```python
from build123d import *

# Parameters (mm, degrees)
BOSS_EXTRUDE1_DEPTH = 3.175
CUT_EXTRUDE1_REACH  = 116.795
SKETCH2_R           = 1.5875


with BuildPart() as part:
    # Sketch1 → Boss-Extrude1 (new body)
    with BuildSketch(Plane.XY):
        Polygon((0, 0), (0, 53.34), (-101.6, 53.34), (-87.988181024, -50.8), align=None)
    extrude(amount=BOSS_EXTRUDE1_DEPTH)

    # Sketch2 → Cut-Extrude1 (cut, up to next)
    with BuildSketch(Plane(origin=(0, 0, 0), x_dir=(-1, 0, 0), z_dir=(0, 0, -1)), mode=Mode.PRIVATE) as cut_extrude1_sk1:
        with Locations((12.7, 40.64)):
            Circle(SKETCH2_R)
    cut_extrude1_tool1 = extrude(cut_extrude1_sk1.sketch, amount=-CUT_EXTRUDE1_REACH, mode=Mode.PRIVATE) & part.part
    # Sketch2 → Cut-Extrude1 (cut, up to next)
    with BuildSketch(Plane(origin=(0, 0, 0), x_dir=(-1, 0, 0), z_dir=(0, 0, -1)), mode=Mode.PRIVATE) as cut_extrude1_sk2:
        with Locations((31.75, 40.64)):
            Circle(SKETCH2_R)
    cut_extrude1_tool2 = extrude(cut_extrude1_sk2.sketch, amount=-CUT_EXTRUDE1_REACH, mode=Mode.PRIVATE) & part.part
    # Sketch2 → Cut-Extrude1 (cut, up to next)
    with BuildSketch(Plane(origin=(0, 0, 0), x_dir=(-1, 0, 0), z_dir=(0, 0, -1)), mode=Mode.PRIVATE) as cut_extrude1_sk3:
        with Locations((50.8, 40.64)):
            Circle(SKETCH2_R)
    cut_extrude1_tool3 = extrude(cut_extrude1_sk3.sketch, amount=-CUT_EXTRUDE1_REACH, mode=Mode.PRIVATE) & part.part
    # Sketch2 → Cut-Extrude1 (cut, up to next)
    with BuildSketch(Plane(origin=(0, 0, 0), x_dir=(-1, 0, 0), z_dir=(0, 0, -1)), mode=Mode.PRIVATE) as cut_extrude1_sk4:
        with Locations((69.85, 40.64)):
            Circle(SKETCH2_R)
    cut_extrude1_tool4 = extrude(cut_extrude1_sk4.sketch, amount=-CUT_EXTRUDE1_REACH, mode=Mode.PRIVATE) & part.part
    # Sketch2 → Cut-Extrude1 (cut, up to next)
    with BuildSketch(Plane(origin=(0, 0, 0), x_dir=(-1, 0, 0), z_dir=(0, 0, -1)), mode=Mode.PRIVATE) as cut_extrude1_sk5:
        with Locations((88.9, 40.64)):
            Circle(SKETCH2_R)
    cut_extrude1_tool5 = extrude(cut_extrude1_sk5.sketch, amount=-CUT_EXTRUDE1_REACH, mode=Mode.PRIVATE) & part.part
    # Sketch2 → Cut-Extrude1 (cut, up to next)
    with BuildSketch(Plane(origin=(0, 0, 0), x_dir=(-1, 0, 0), z_dir=(0, 0, -1)), mode=Mode.PRIVATE) as cut_extrude1_sk6:
        with Locations((11.903880744, 8.025962948)):
            Circle(SKETCH2_R)
    cut_extrude1_tool6 = extrude(cut_extrude1_sk6.sketch, amount=-CUT_EXTRUDE1_REACH, mode=Mode.PRIVATE) & part.part
    # Sketch2 → Cut-Extrude1 (cut, up to next)
    with BuildSketch(Plane(origin=(0, 0, 0), x_dir=(-1, 0, 0), z_dir=(0, 0, -1)), mode=Mode.PRIVATE) as cut_extrude1_sk7:
        with Locations((28.401664686, -1.499037052)):
            Circle(SKETCH2_R)
    cut_extrude1_tool7 = extrude(cut_extrude1_sk7.sketch, amount=-CUT_EXTRUDE1_REACH, mode=Mode.PRIVATE) & part.part
    # Sketch2 → Cut-Extrude1 (cut, up to next)
    with BuildSketch(Plane(origin=(0, 0, 0), x_dir=(-1, 0, 0), z_dir=(0, 0, -1)), mode=Mode.PRIVATE) as cut_extrude1_sk8:
        with Locations((44.899448628, -11.024037052)):
            Circle(SKETCH2_R)
    cut_extrude1_tool8 = extrude(cut_extrude1_sk8.sketch, amount=-CUT_EXTRUDE1_REACH, mode=Mode.PRIVATE) & part.part
    # Sketch2 → Cut-Extrude1 (cut, up to next)
    with BuildSketch(Plane(origin=(0, 0, 0), x_dir=(-1, 0, 0), z_dir=(0, 0, -1)), mode=Mode.PRIVATE) as cut_extrude1_sk9:
        with Locations((61.39723257, -20.549037052)):
            Circle(SKETCH2_R)
    cut_extrude1_tool9 = extrude(cut_extrude1_sk9.sketch, amount=-CUT_EXTRUDE1_REACH, mode=Mode.PRIVATE) & part.part
    # Sketch2 → Cut-Extrude1 (cut, up to next)
    with BuildSketch(Plane(origin=(0, 0, 0), x_dir=(-1, 0, 0), z_dir=(0, 0, -1)), mode=Mode.PRIVATE) as cut_extrude1_sk10:
        with Locations((77.895016512, -30.074037052)):
            Circle(SKETCH2_R)
    cut_extrude1_tool10 = extrude(cut_extrude1_sk10.sketch, amount=-CUT_EXTRUDE1_REACH, mode=Mode.PRIVATE) & part.part
    add(cut_extrude1_tool1.solids().sort_by_distance((-12.7, 40.64, 0))[0], mode=Mode.SUBTRACT)
    add(cut_extrude1_tool2.solids().sort_by_distance((-31.75, 40.64, 0))[0], mode=Mode.SUBTRACT)
    add(cut_extrude1_tool3.solids().sort_by_distance((-50.8, 40.64, 0))[0], mode=Mode.SUBTRACT)
    add(cut_extrude1_tool4.solids().sort_by_distance((-69.85, 40.64, 0))[0], mode=Mode.SUBTRACT)
    add(cut_extrude1_tool5.solids().sort_by_distance((-88.9, 40.64, 0))[0], mode=Mode.SUBTRACT)
    add(cut_extrude1_tool6.solids().sort_by_distance((-11.903881, 8.025963, 0))[0], mode=Mode.SUBTRACT)
    add(cut_extrude1_tool7.solids().sort_by_distance((-28.401665, -1.499037, 0))[0], mode=Mode.SUBTRACT)
    add(cut_extrude1_tool8.solids().sort_by_distance((-44.899449, -11.024037, 0))[0], mode=Mode.SUBTRACT)
    add(cut_extrude1_tool9.solids().sort_by_distance((-61.397233, -20.549037, 0))[0], mode=Mode.SUBTRACT)
    add(cut_extrude1_tool10.solids().sort_by_distance((-77.895017, -30.074037, 0))[0], mode=Mode.SUBTRACT)


solid = part.part
```
CAD build for the part. Positions are in the model's coordinates, mm. Give positions to 0.01 mm unless a question says otherwise; leave off trailing zeros. Order: outer loops, then holes, each group sorted by start corner. A loop starts at its lowest first (then second) coordinate and runs counter-clockwise, first axis right, second up. Notation, with made-up numbers: M 89.5,67.25 L 98.5,67.25 A4 ccw 98.5,73.25 Z; hole C 31.5,29.5 d6. An arc over 180 degrees is marked long. Put each result on its own line as item: value. Start each with the question number.
(1) Flat gauge pins, fed straight in: pin 1 Ø1 at (y, z) = (13.5, 1.5) entering from -X; pin 2 Ø5 at (x, y) = (-28.4, -1.5) entering from +Z (3 decimals); pin 3 Ø1 at (y, z) = (13, 1.5) entering from -X. Where does each tip first touch, or does it go through?
(2) Saw through at C-C, the plane z = 1. Give the number of separate pieces and of enclosed holes in the cut face, then the cut area to 3 significant figures.
(3) Saw through at D-D, the plane x = -69.85. Write the cut outline in (y, z) (1 decimal).
(4) Saw through at B-B, the plane y = 40.64. Write the cut outline in (x, z) (1 decimal).
(5) Drill centre lines: line 1 along Y through (x, z) = (-12, 1.9); line 2 along Y through (x, z) = (-12.7, 1.25); line 3 along Y through (x, z) = (-70, 2.2). Where is each one in solid material? Low to high.
(6) Mould opens along X. For faces 1 (the flat face through (-52, 14, 0)), 2 (the flat face through (-94.89, 2, 1.57)), 3 (the cylindrical face through (-90.366, 40.032, 1.565)), 4 (the cylindrical face through (-10.644, 7.06, 1.565)) say: +X half, -X half, draft (parallel to the pull), parting line (faces both ways), or undercut.
(7) Saw through at A-A, the plane x = -31.75. Write the cut outline in (y, z) (1 decimal).
Check result:
1. pin 1: stops at x = -96.46
1. pin 2: stops at z = 3.175
1. pin 3: stops at x = -96.39
2. separate pieces: 1
2. enclosed holes: 10
2. area: 7,560 mm2
3. outline: M -40.3,0 L 39.1,0 L 39.1,3.2 L -40.3,3.2 Z; M 42.2,0 L 53.3,0 L 53.3,3.2 L 42.2,3.2 Z
4. outline: M -99.9,0 L -90.5,0 L -90.5,3.2 L -99.9,3.2 Z; M -87.3,0 L -71.4,0 L -71.4,3.2 L -87.3,3.2 Z; M -68.3,0 L -52.4,0 L -52.4,3.2 L -68.3,3.2 Z; M -49.2,0 L -33.3,0 L -33.3,3.2 L -49.2,3.2 Z; M -30.2,0 L -14.3,0 L -14.3,3.2 L -30.2,3.2 Z; M -11.1,0 L 0,0 L 0,3.2 L -11.1,3.2 Z
5. line 1: y = -6.93 to 6.44, 9.61 to 39.22, 42.06 to 53.34
5. line 2: y = -7.33 to 6.65, 9.4 to 39.05, 42.23 to 53.34
5. line 3: y = -40.41 to 39.06, 42.22 to 53.34
6. face 1: draft
6. face 2: -X half
6. face 3: undercut
6. face 4: undercut
7. outline: M -18.3,0 L 39.1,0 L 39.1,3.2 L -18.3,3.2 Z; M 42.2,0 L 53.3,0 L 53.3,3.2 L 42.2,3.2 Z
